For this review, take the finished solid that the model builds, in its own axes (mm). Round coordinates to 2 decimals unless told otherwise and drop trailing zeros. Order: outer loops, then holes, each group sorted by start corner. A loop starts at its lowest first (then second) coordinate and runs counter-clockwise, first axis right, second up.
from build123d import *

# Parameters (mm, degrees)
PLATE_DEPTH                  = 3
SKETCH4_R                    = 3
PIVOT_HOLES_ARM_DEPTH        = 4
SKETCH5_R                    = 2.05
CHASSIS_HOLES_DEPTH          = 4
CSK_FOR_M4_SFHCS1_AT_2_COUNT = 2
CSK_FOR_M4_SFHCS1_AT_2_PITCH = 54.708317466
CSK_FOR_M4_SFHCS1_AT_3_COUNT = 2
CSK_FOR_M4_SFHCS1_AT_3_PITCH = 165.871053731
CSK_FOR_M4_SFHCS1_AT_4_COUNT = 2
CSK_FOR_M4_SFHCS1_AT_4_PITCH = 187.072959568


with BuildPart() as part:
    # Sketch2 → Plate (new body)
    with BuildSketch(Plane.XY):
        with BuildLine():
            Line((-80, -12), (80, -12))
            Line((80, -12), (109.503808991, -7))
            ThreePointArc((109.503808991, -7), (113.481492527, -1.271406135), (111.490110497, 5.412391557))
            Line((111.490110497, 5.412391557), (61.490110497, 60.412391557))
            ThreePointArc((61.490110497, 60.412391557), (54.517770463, 62.981349031), (48.414233747, 58.743435912))
            Line((48.414233747, 58.743435912), (40.824196955, 44.302662586))
            ThreePointArc((40.824196955, 44.302662586), (37.862458518, 41.159163218), (33.701950918, 40))
            Line((33.701950918, 40), (-33.701950918, 40))
            ThreePointArc((-33.701950918, 40), (-37.862458518, 41.159163218), (-40.824196955, 44.302662586))
            Line((-40.824196955, 44.302662586), (-48.414233747, 58.743435912))
            ThreePointArc((-48.414233747, 58.743435912), (-54.517770463, 62.981349031), (-61.490110497, 60.412391557))
            Line((-61.490110497, 60.412391557), (-111.490110497, 5.412391557))
            ThreePointArc((-111.490110497, 5.412391557), (-113.481492527, -1.271406135), (-109.503808991, -7))
            Line((-109.503808991, -7), (-80, -12))
        make_face()
    extrude(amount=PLATE_DEPTH)

    # Sketch4 → Pivot holes (arm) (cut, through all)
    with BuildSketch(Plane.XY):
        with Locations((105.536479784, 0)):
            Circle(SKETCH4_R)
        with Locations((55.536479784, 10)):
            Circle(SKETCH4_R)
        with Locations((55.536479784, 55)):
            Circle(SKETCH4_R)
        with Locations((-105.536479784, 0)):
            Circle(SKETCH4_R)
        with Locations((-55.536479784, 10)):
            Circle(SKETCH4_R)
        with Locations((-55.536479784, 55)):
            Circle(SKETCH4_R)
        with Locations((-21.998408138, 15.585494631)):
            Circle(SKETCH4_R)
        with Locations((21.998408138, 15.585494631)):
            Circle(SKETCH4_R)
    extrude(amount=PIVOT_HOLES_ARM_DEPTH, mode=Mode.SUBTRACT)

    # Sketch5 → Chassis holes (cut, through all)
    with BuildSketch(Plane.XY.offset(3)):
        with Locations((-19.5, -2)):
            Circle(SKETCH5_R)
        with Locations((19.5, -2)):
            Circle(SKETCH5_R)
    extrude(amount=-CHASSIS_HOLES_DEPTH, mode=Mode.SUBTRACT)

    # Sketch7 → CSK for M4 SFHCS1 (revolve, cut)
    with BuildSketch(Plane(origin=(93.536479784, -2, 3), x_dir=(0, -1, 0), z_dir=(1, 0, 0))):
        Polygon((0, 0), (0, 3), (2.25, 3), (2.25, 2.23), (4.48, 0), align=None)
    csk_for_m4_sfhcs1 = revolve(axis=Axis((93.536479784, -2, 9.35), (0, 0, -1)), mode=Mode.SUBTRACT)

    # CSK for M4 SFHCS1 at 2: CSK for M4 SFHCS1 ×2
    with Locations(*[Vector(-0.511805175, 0.859101544, 0) * (i * CSK_FOR_M4_SFHCS1_AT_2_PITCH) for i in range(1, CSK_FOR_M4_SFHCS1_AT_2_COUNT)]):
        add(csk_for_m4_sfhcs1, mode=Mode.SUBTRACT)

    # CSK for M4 SFHCS1 at 3: CSK for M4 SFHCS1 ×2
    with Locations(*[Vector(-0.95901579, 0.283352634, 0) * (i * CSK_FOR_M4_SFHCS1_AT_3_PITCH) for i in range(1, CSK_FOR_M4_SFHCS1_AT_3_COUNT)]):
        add(csk_for_m4_sfhcs1, mode=Mode.SUBTRACT)

    # CSK for M4 SFHCS1 at 4: CSK for M4 SFHCS1 ×2
    with Locations(*[(-i * CSK_FOR_M4_SFHCS1_AT_4_PITCH, 0, 0) for i in range(1, CSK_FOR_M4_SFHCS1_AT_4_COUNT)]):
        add(csk_for_m4_sfhcs1, mode=Mode.SUBTRACT)


solid = part.part
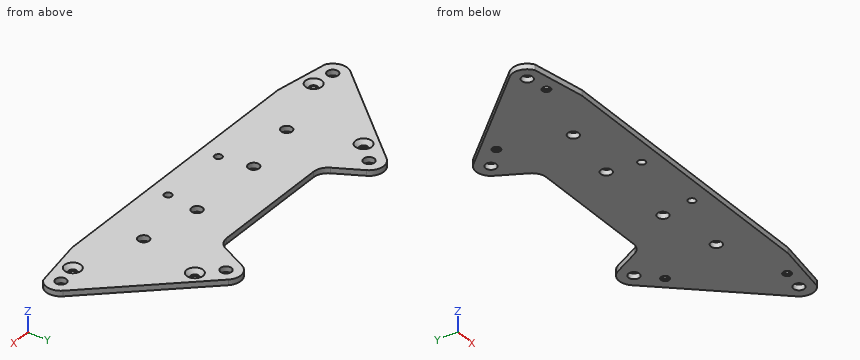
(1) Add section A-A on y = 10. Give the boundary of the cut face in (x, z), plus the area to 3 significant figures.
(2) Clearance check with flat-ended pins moving along their axes: P1, Ø4, axis at x = -65.54, y = 45, coming from the +Z side; P2, Ø0.9, axis at x = -15.5, z = 1.5, coming from the +Y side; P3, Ø7, axis at x = -105.54, y = 0, coming from the -Z side; P4, Ø6, axis at x = 65.54, y = 45, coming from the +Z side. State where each tip first meets the part, or that it passes through.
(3) Add section C-C on x = 55. Give the boundary of the cut face in (y, z).
(4) Add section D-D on x = 3.5. Give the boundary of the cut face in (y, z), plus the area to 3 significant figures.
(5) Wall thickness on L1, parallel to X at y = 57, z = 1.6; L2, parallel to X at y = 2.5, z = 0.45; L3, parallel to Y at x = -12, z = 1.95: over which ranges is each line inside the solid? List them lowest first.
(6) Add section B-B on z = 2.25. Count the separate pieces of the cut face and the enclosed holes in it, plus the area to 3 significant figures.
Here are the results:
1. outline: (-107.32, 0) - (-58.54, 0) - (-58.54, 3) - (-107.32, 3) - close; (-52.54, 0) - (52.54, 0) - (52.54, 3) - (-52.54, 3) - close; (58.54, 0) - (107.32, 0) - (107.32, 3) - (58.54, 3) - close
1. area: 608 mm2
2. P1: passes through
2. P2: stops at y = 40
2. P3: stops at z = 0
2. P4: stops at z = 1.52
3. outline: (-12, 0) - (7.05, 0) - (7.05, 3) - (-12, 3) - close; (12.95, 0) - (52.05, 0) - (52.05, 3) - (12.95, 3) - close; (57.95, 0) - (63.03, 0) - (63.03, 3) - (57.95, 3) - close
4. outline: (-12, 0) - (40, 0) - (40, 3) - (-12, 3) - close
4. area: 156 mm2
5. L1: x = -64.59 to -57.77, -53.3 to -47.5, 47.5 to 53.3, 57.77 to 64.59
5. L2: x = -113.18 to -107.19, -103.88 to 103.88, 107.19 to 113.18
5. L3: y = -12 to 40
6. separate pieces: 1
6. enclosed holes: 14
6. area: 11,100 mm2
